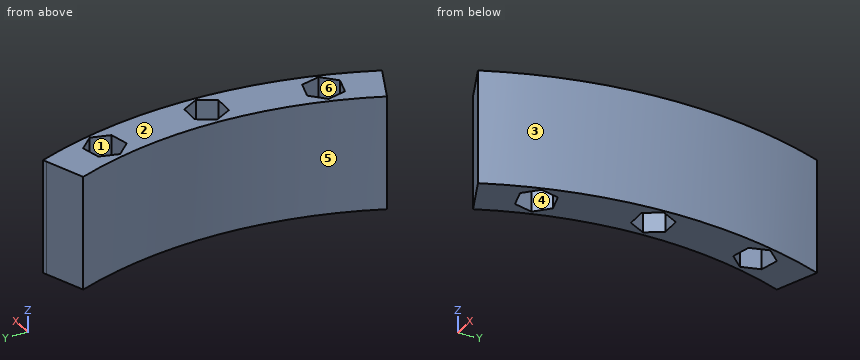
from build123d import *

# Parameters (mm, degrees)
BOSS_EXTRUDE1_START = 0.01
BOSS_EXTRUDE1_DEPTH = 21.8


with BuildPart() as part:
    # Sketch1 → Boss-Extrude1 (new body)
    with BuildSketch(Plane.XY.offset(BOSS_EXTRUDE1_START)):
        with BuildLine():
            Line((77.199593807, -31.819376425), (69.803225538, -28.770813414))
            ThreePointArc((69.803225538, -28.770813414), (75.5, 0), (69.803225538, 28.770813414))
            Line((69.803225538, 28.770813414), (77.199593807, 31.819376425))
            Line((77.199593807, 31.819376425), (77.893003332, 32.105179208))
            ThreePointArc((77.893003332, 32.105179208), (84.25, 0), (77.893003332, -32.105179208))
            Line((77.893003332, -32.105179208), (77.199593807, -31.819376425))
        make_face()
        Polygon((76.24722325, 0), (78.123611625, -3.25), (81.876388375, -3.25), (83.75277675, 0), (81.876388375, 3.25), (78.123611625, 3.25), align=None, mode=Mode.SUBTRACT)
        Polygon((79.927679991, 18.05190972), (76.302776008, 17.080619625), (73.64916212, 19.734233513), (74.620452215, 23.359137496), (78.245356198, 24.330427591), (80.898970086, 21.676813703), align=None, mode=Mode.SUBTRACT)
        Polygon((74.620452215, -23.359137496), (78.245356198, -24.330427591), (80.898970086, -21.676813703), (79.927679991, -18.05190972), (76.302776008, -17.080619625), (73.64916212, -19.734233513), align=None, mode=Mode.SUBTRACT)
    extrude(amount=BOSS_EXTRUDE1_DEPTH)


solid = part.part
Geometry: final body of the model. Coordinates: model frame, mm. Face numbers are marked on the shaded views. A direction names the side the tool comes from. Coordinates: 2 decimals unless noted, no trailing zeros. Order: outer loops, then holes, each group sorted by start corner. A loop starts at its lowest first (then second) coordinate and runs counter-clockwise, first axis right, second up. Notation, with made-up numbers: M -6.5,22.5 L 48.5,22.5 A13 cw 48.5,31.5 Z; hole C 57,-16.75 d6. An arc over 180 degrees is marked long. One line per question, with ' | ' between items. Start each with the question number.
Item 1: Ray query, probe 1 along X at (y, z) = (-22, 16); probe 2 along X at (y, z) = (-1, 13.75); probe 3 along X at (y, z) = (-28, 9.75). Return the intervals inside material, ascending. Write a range as [from, to].
Item 2: Set-up query: the marked faces 5 and 6. Return all of +Z, -Z, +X, -X, +Y, -Y with unobstructed straight access to the full face (end or side cutting, diameter ignored); none if empty.
Item 3: Cut plane A-A, the plane z = 16.5. Return the cut outline in (x, y), then the cut area to 3 significant figures.
Item 4: Cut plane B-B, the plane y = -1.5. Return the cut outline in (x, z), then the cut area to 3 significant figures.
Item 5: Draft query along X for the marked faces 1, 2, 3 and 4. Return one class per face: released by +X, released by -X, zero draft, split by the parting line, or undercut.
Item 6: Cut plane D-D, the plane y = -25.5. Return the cut outline in (x, z).
Item 7: Pin query (flat end, axial travel): pin 1 Ø1 at (y, z) = (-4, 14.5) entering from -X; pin 2 Ø1.5 at (y, z) = (-23.5, 14) entering from -X; pin 3 Ø10 at (y, z) = (23, 17.5) entering from +X. Return the tip coordinate at first contact, or that it passes through.
Item 8: Cut plane C-C, the plane x = 72. Return the cut outline in (y, z).
A:
1) probe 1: x = [72.22, 74.26], [80.58, 81.33] | probe 2: x = [75.49, 76.82], [83.18, 84.24] | probe 3: x = [70.12, 79.46]
2) face 5: +Z, -Z, -X | face 6: +Z, -Z
3) outline: M 69.8,-28.77 L 77.89,-32.11 A84.25 ccw 77.89,32.11 L 69.8,28.77 A75.5 cw Z; hole M 73.65,-19.73 L 74.62,-23.36 L 78.25,-24.33 L 80.9,-21.68 L 79.93,-18.05 L 76.3,-17.08 Z; hole M 73.65,19.73 L 76.3,17.08 L 79.93,18.05 L 80.9,21.68 L 78.25,24.33 L 74.62,23.36 Z; hole M 76.25,0 L 78.12,-3.25 L 81.88,-3.25 L 83.75,0 L 81.88,3.25 L 78.12,3.25 Z | area: 437 mm2
4) outline: M 75.49,0.01 L 77.11,0.01 L 77.11,21.81 L 75.49,21.81 Z; M 82.89,0.01 L 84.24,0.01 L 84.24,21.81 L 82.89,21.81 Z | area: 64.9 mm2
5) face 1: undercut | face 2: zero draft | face 3: released by +X | face 4: undercut
6) outline: M 71.06,0.01 L 80.3,0.01 L 80.3,21.81 L 71.06,21.81 Z
7) pin 1: stops at x = 75.37 | pin 2: stops at x = 71.5 | pin 3: stops at x = 82.3
8) outline: M -29.68,0.01 L -22.72,0.01 L -22.72,21.81 L -29.68,21.81 Z; M 22.72,0.01 L 29.68,0.01 L 29.68,21.81 L 22.72,21.81 Z
